Input: part model. Units: mm. Frame: model coordinates. Coordinates: 2 decimals unless noted, no trailing zeros. Write each loop counter-clockwise with the first axis right and the second up, starting at its lowest first coordinate (ties: lowest second). Pieces come first, ordered by that corner, then holes. Notation, with made-up numbers: (76.25, -30) - (80.25, -30) arc R26 cw to (80.25, 4) - close; hole circle Ø5 at (34.5, 54). An arc over 180 degrees is marked (long way). Put each result on its own line as item: value. Start each with the question number.
1. Line query: line 1 (X direction, y = 1.5, z = -5.25); line 2 (Z direction, x = 27.5, y = 21); line 3 (Y direction, x = 27.5, z = -5). Output: solid intervals per line, ascending.
2. Pin query (flat end, axial travel): pin 1 (0.9 mm diameter, centred on x = 63.5, z = -4.5, fed in from +Y); pin 2 (4 mm diameter, centred on x = 148.5, z = -6.5, fed in from -Y); pin 3 (2.5 mm diameter, centred on x = -122.62, z = -5, fed in from -Y). Return the tip coordinate at first contact, or that it passes through.
3. Cut plane A-A, the plane x = 103.5. Return loops of the section in (y, z).
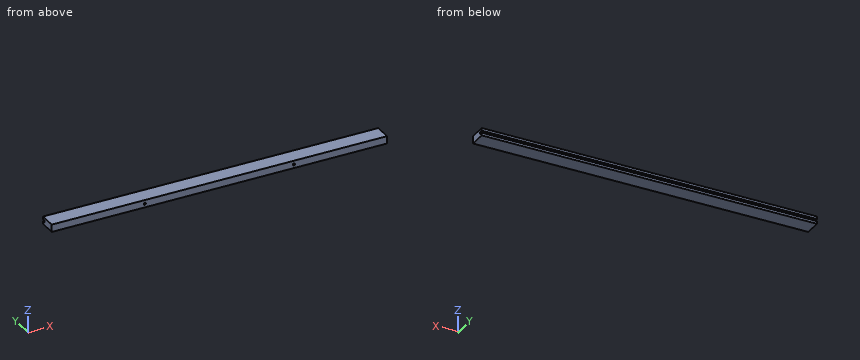
from build123d import *

# Parameters (mm, degrees)
SZKIC1_W                       = 450
SZKIC1_H                       = 10
DODANIE_WYCI_GNI_CIE1_DEPTH    = 22
SZKIC2_W                       = 450
SZKIC2_H                       = 3
WYTNIJ_WYCI_GNI_CIE1_DEPTH     = 4
OTWORY_USTALAJ_CE_3_0MM1_D     = 3
OTWORY_USTALAJ_CE_3_0MM1_DEPTH = 10
OTWORY_USTALAJ_CE_3_0MM1_TIP   = 0.901290929


with BuildPart() as part:
    # Szkic1 → Dodanie-wyciągnięcie1 (new body)
    with BuildSketch(Plane(origin=(0, 0, 0), x_dir=(1, 0, 0), z_dir=(0, 1, 0))):
        with Locations((-22.623576347, 5)):
            Rectangle(SZKIC1_W, SZKIC1_H)
    extrude(amount=DODANIE_WYCI_GNI_CIE1_DEPTH)

    # Szkic2 → Wytnij-wyciągnięcie1 (cut)
    with BuildSketch(Plane(origin=(0, 22, 0), x_dir=(1, 0, 0), z_dir=(0, 1, 0))):
        with Locations((-22.623576347, 5)):
            Rectangle(SZKIC2_W, SZKIC2_H)
    extrude(amount=-WYTNIJ_WYCI_GNI_CIE1_DEPTH, mode=Mode.SUBTRACT)

    # Otwory ustalające Ø3.0mm1
    with Locations(Plane(origin=(0, 0, 0), x_dir=(-1, 0, 0), z_dir=(0, -1, 0))):
        with Locations((-77.376423653, 5), (122.623576347, 5)):
            Hole(OTWORY_USTALAJ_CE_3_0MM1_D / 2, depth=OTWORY_USTALAJ_CE_3_0MM1_DEPTH)
            with Locations((0, 0, -(OTWORY_USTALAJ_CE_3_0MM1_DEPTH + OTWORY_USTALAJ_CE_3_0MM1_TIP / 2))):  # 118° drill point
                Cone(0, OTWORY_USTALAJ_CE_3_0MM1_D / 2, OTWORY_USTALAJ_CE_3_0MM1_TIP, mode=Mode.SUBTRACT)


solid = part.part
Report:
1. line 1: x = -247.62 to -124.1, -121.14 to 75.9, 78.86 to 202.38
1. line 2: z = -10 to -6.5, -3.5 to 0
1. line 3: y = 0 to 18
2. pin 1: stops at y = 18
2. pin 2: stops at y = 0
2. pin 3: stops at y = 10.15
3. outline: (0, -10) - (22, -10) - (22, -6.5) - (18, -6.5) - (18, -3.5) - (22, -3.5) - (22, 0) - (0, 0) - close
